Autodesk Inventor part; units mm, degrees
ref_plane "YZ Plane" through (0, 0, 0) normal (1, 0, 0) x (0, 1, 0)
ref_plane "XZ Plane" through (0, 0, 0) normal (0, 1, 0) x (-1, 0, 0)
ref_plane "XY Plane" through (0, 0, 0) normal (0, 0, 1) x (1, 0, 0)
sketch "Sketch1" plane through (0, 0, 0) normal (0, 0, 1) x (1, 0, 0)
  line L0 (0, 0) -> (25.4, 0)
  line L1 (25.4, 0) -> (25.4, 25.4)
  line L2 (25.4, 25.4) -> (0, 25.4)
  line L3 (0, 25.4) -> (0, 0)
  line L4 (3.175, 22.225) -> (22.225, 22.225)
  line L5 (22.225, 22.225) -> (22.225, 3.175)
  line L6 (22.225, 3.175) -> (3.175, 3.175)
  line L7 (3.175, 3.175) -> (3.175, 22.225)
  dimension "d0" = 25.4
  dimension "d1" = 25.4
  dimension "d2" = 3.175
extrude "Extrusion1" add sketch "Sketch1" along normal blind 635
sketch "Sketch2" plane through (25.4, 0, 0) normal (1, 0, 0) x (0, 0, -1)
  line L0 (0, 0) -> (0, 25.4) construction
  line L1 (0, 25.4) -> (0, 18.7198) construction
  line L2 (0, 25.4) -> (0, 21.7678) construction
  line L3 (0, 22.225) -> (-635, 22.225) construction
  line L4 (0, 21.7678) -> (-76.2, 21.7678) construction
  line L5 (-76.2, 21.7678) -> (-177.8, 21.7678) construction
  line L6 (-177.8, 21.7678) -> (-279.4, 21.7678) construction
  line L7 (-279.4, 21.7678) -> (-381, 21.7678) construction
  line L8 (-381, 21.7678) -> (-482.6, 21.7678) construction
  line L9 (-482.6, 21.7678) -> (-584.2, 21.7678) construction
  circle A0 centre (-76.2, 21.7678) radius 1.3208
  circle A1 centre (-177.8, 21.7678) radius 1.3208
  circle A2 centre (-279.4, 21.7678) radius 1.3208
  circle A3 centre (-381, 21.7678) radius 1.3208
  circle A4 centre (-482.6, 21.7678) radius 1.3208
  circle A5 centre (-584.2, 21.7678) radius 1.3208
  dimension "d5" = 6.6802
  dimension "d6" = 3.6322
  dimension "d8" = 76.2
  dimension "d9" = 101.6
  dimension "d11" = 101.6
  dimension "d12" = 101.6
  dimension "d13" = 101.6
  dimension "d14" = 101.6
  dimension "d15" = 2.6416
extrude "Extrusion2" cut sketch "Sketch2" against normal blind 635
sketch "Sketch3" plane through (0, 0, 635) normal (0, 0, 1) x (1, 0, 0)
  line L0 (3.175, 3.175) -> (3.175, 22.225)
  line L1 (3.175, 22.225) -> (22.225, 22.225)
  line L2 (22.225, 22.225) -> (22.225, 42.4073)
  line L3 (22.225, 42.4073) -> (3.175, 42.4073)
  line L4 (3.175, 42.4073) -> (3.175, 22.225)
  point P0 (0, 0)
  dimension "d18" = 19.05
extrude "Extrusion3" cut sketch "Sketch3" against normal blind 635
sketch "Sketch4" plane through (25.4, 0, 0) normal (1, 0, 0) x (0, 0, -1)
  line L0 (0, 25.4) -> (0, 0)
  line L1 (0, 12.7) -> (-12.7, 12.7) construction
  line L2 (0, 12.7) -> (12.7, 12.7) construction
  circle A0 centre (-12.7, 12.7) radius 2.5797
  dimension "d21" = 12.7
  dimension "d22" = 180
  dimension "d23" = 5.1594
extrude "Extrusion4" cut sketch "Sketch4" against normal blind 635
sketch "Sketch5" plane through (0, 0, 0) normal (0, -1, 0) x (1, 0, 0)
  line L0 (0, 0) -> (25.4, 0) construction
  line L1 (12.7, 0) -> (12.7, 12.7) construction
  line L2 (12.7, 0) -> (25.4, 0) construction
  circle A0 centre (12.7, 12.7) radius 2.5797
  dimension "d26" = 12.7
  dimension "d27" = 90
  dimension "d28" = 5.1594
extrude "Extrusion6" cut sketch "Sketch5" against normal blind 635
properties part number "1x1 U-Channel"
Work out the finished part from the listing and answer in its coordinate system (mm). A direction names the side the tool comes from. Round coordinates to 2 decimals unless told otherwise and drop trailing zeros. Loops run counter-clockwise (first coordinate to the right, second up) from the corner with the lowest first, then second, coordinate; pieces in that order, holes last. Notation, with made-up numbers: M -25,-25.5 L -3,-25.5 A30 ccw -3,9.5 Z; hole C 64.25,62 d3. An arc over 180 degrees is marked long. One line per question, with ' | ' between items.
Q1. Consider line 1 along X through (y, z) = (18.25, 222) (3 decimals); line 2 along Y through (x, z) = (1, 381); line 3 along Y through (x, z) = (9.75, 531.5) (3 decimals). Determine where each line is inside the solid, lowest interval first. Write a range as from..to.
Conclusion:
line 1: x = 0..3.175, 22.225..25.4 | line 2: y = 0..20.45, 23.09..25.4 | line 3: y = 0..3.175
Q2. The mould has two halves that part along X. Classify faces 3 (the flat face through (0, 13, 313)), 4 (the flat face through (13, 0, 313)), 5 (the flat face through (13, 3.175, 313)), 6 (the flat face through (3.175, 14, 322)): +X half, -X half, draft (parallel to the pull), parting line (faces both ways), or undercut.
Conclusion:
face 3: -X half | face 4: draft | face 5: undercut | face 6: undercut
Q3. A tool of negligible diameter and unlimited length cuts with its end or side. For faces 1 (the flat face through (22.225, 14, 313)), 2 (the flat face through (25.4, 13, 313)), from which of +Z, -Z, +X, -X, +Y, -Y can it reach the whole face along a straight path? Write none if from no direction.
Conclusion:
face 1: +Z, -Z, +Y | face 2: +Z, -Z, +X, +Y, -Y
Q4. Each of these flat-tipped pins is pushed along its axis until it touches: pin 1 Ø3 at (y, z) = (21.77, 381) entering from -X; pin 2 Ø15 at (x, z) = (11, 430.5) entering from +Y (3 decimals). Where does it stop, or does it pass through?
Conclusion:
pin 1: stops at x = 0 | pin 2: stops at y = 3.175
Q5. Find section A-A, the plane z = 527. Give the vertices of the cut face in (x, y) (3 decimals), then the cut area to 3 significant figures.
Conclusion:
outline: M 0,0 L 25.4,0 L 25.4,25.4 L 22.225,25.4 L 22.225,3.175 L 3.175,3.175 L 3.175,25.4 L 0,25.4 Z | area: 222 mm2
